from build123d import *

# Parameters (mm, degrees)
SKETCH1_W            = 60
SKETCH1_H            = 20
BOSS_EXTRUDE1_DEPTH  = 3
FILLET1_R            = 10
SKETCH36_R           = 7.1
BOSS_EXTRUDE15_DEPTH = 2
SKETCH37_R           = 9.2
BOSS_EXTRUDE16_DEPTH = 2
SKETCH39_R           = 7.1
BOSS_EXTRUDE18_DEPTH = 2
SKETCH40_R           = 9.2
BOSS_EXTRUDE19_DEPTH = 2
SKETCH41_R           = 7.1
BOSS_EXTRUDE20_DEPTH = 2
SKETCH42_R           = 4
CUT_EXTRUDE5_DEPTH   = 13
SKETCH43_R           = 2.75
CUT_EXTRUDE6_DEPTH   = 3


with BuildPart() as part:
    # Sketch1 → Boss-Extrude1 (new body)
    with BuildSketch(Plane(origin=(0, 0, 0), x_dir=(1, 0, 0), z_dir=(0, 1, 0))):
        Rectangle(SKETCH1_W, SKETCH1_H)
    extrude(amount=BOSS_EXTRUDE1_DEPTH)

    # Fillet1
    fillet1_edges = [part.edges().sort_by_distance(p)[0] for p in [
        (30, 1.5, -10),
        (30, 1.5, 10),
        (-30, 1.5, 10),
        (-30, 1.5, -10),
    ]]
    fillet(fillet1_edges, radius=FILLET1_R - 0.0001)  # a hair under: the kernel refuses the full size

    # Sketch36 → Boss-Extrude15 (add)
    with BuildSketch(Plane(origin=(0, 3, 0), x_dir=(1, 0, 0), z_dir=(0, 1, 0))):
        with Locations(Location((0, 0, 0), (0, 0, 90))):
            Circle(SKETCH36_R)
    extrude(amount=BOSS_EXTRUDE15_DEPTH)

    # Sketch37 → Boss-Extrude16 (add)
    with BuildSketch(Plane(origin=(0, 5, 0), x_dir=(1, 0, 0), z_dir=(0, 1, 0))):
        with Locations(Location((0, 0, 0), (0, 0, 270))):
            Circle(SKETCH37_R)
    extrude(amount=BOSS_EXTRUDE16_DEPTH)

    # Sketch39 → Boss-Extrude18 (add)
    with BuildSketch(Plane(origin=(0, 7, 0), x_dir=(1, 0, 0), z_dir=(0, 1, 0))):
        with Locations(Location((0, 0, 0), (0, 0, 90))):
            Circle(SKETCH39_R)
    extrude(amount=BOSS_EXTRUDE18_DEPTH)

    # Sketch40 → Boss-Extrude19 (add)
    with BuildSketch(Plane(origin=(0, 9, 0), x_dir=(1, 0, 0), z_dir=(0, 1, 0))):
        with Locations(Location((0, 0, 0), (0, 0, 270))):
            Circle(SKETCH40_R)
    extrude(amount=BOSS_EXTRUDE19_DEPTH)

    # Sketch41 → Boss-Extrude20 (add)
    with BuildSketch(Plane(origin=(0, 11, 0), x_dir=(1, 0, 0), z_dir=(0, 1, 0))):
        with Locations(Location((0, 0, 0), (0, 0, 90))):
            Circle(SKETCH41_R)
    extrude(amount=BOSS_EXTRUDE20_DEPTH)

    # Sketch42 → Cut-Extrude5 (cut)
    with BuildSketch(Plane(origin=(0, 13, 0), x_dir=(1, 0, 0), z_dir=(0, 1, 0))):
        with Locations(Location((0, 0, 0), (0, 0, 270))):
            Circle(SKETCH42_R)
    extrude(amount=-CUT_EXTRUDE5_DEPTH, mode=Mode.SUBTRACT)

    # Sketch43 → Cut-Extrude6 (cut)
    with BuildSketch(Plane(origin=(0, 3, 0), x_dir=(1, 0, 0), z_dir=(0, 1, 0))):
        with Locations(Location((-20, 0, 0), (0, 0, 270))):
            Circle(SKETCH43_R)
        with Locations(Location((20, 0, 0), (0, 0, 270))):
            Circle(SKETCH43_R)
    extrude(amount=-CUT_EXTRUDE6_DEPTH, mode=Mode.SUBTRACT)


solid = part.part
Model file for the job. Use its own axes, mm. A direction names the side the tool comes from. Give positions to 0.01 mm unless a question says otherwise; leave off trailing zeros. Loops run counter-clockwise (first coordinate to the right, second up) from the corner with the lowest first, then second, coordinate; pieces in that order, holes last.
1) Saw through at C-C (z = -5.5). Write the cut outline in (x, y), plus the area to 3 significant figures.
2) Saw through at D-D (z = -8). Write the cut outline in (x, y), plus the area to 3 significant figures.
3) Flat gauge pins, fed straight in: pin 1 Ø1.5 at (x, y) = (-5, 7.5) entering from +Z; pin 2 Ø6.5 at (x, z) = (20, 0) entering from +Y; pin 3 Ø4 at (x, z) = (-9.5, -5) entering from +Y. Where does each tip first touch, or does it go through?
4) Saw through at B-B (y = 1.75). Count the separate pieces of the cut face and the enclosed holes in it, plus the area to 3 significant figures.
5) Tool access for faces 4 (the cylindrical face through (2.763, 5.986, 8.775)), 5 (the cylindrical face through (-5.987, 3.986, -3.817)), 6 (the cylindrical face through (27.15, 1.52, -6.99)): list every direction of +Z, -Z, +X, -X, +Y, -Y with a clear straight run to the whole face (end or side of a thin tool).
6) Pull direction Y, two halves, no side cores. Call faces 1 (the flat face through (0, 0, -5)), 2 (the flat face through (0, 1, 10)), 3 (the cylindrical face through (-5.987, 7.986, -3.817)): +Y half, -Y half, draft (parallel to the pull), parting line (faces both ways), or undercut.
7) Wall check: line 1 (X direction, y = 1.4, z = 0); line 2 (Y direction, x = -8, z = -1.5); line 3 (X direction, y = 6, z = 0). Give the ranges that are in metal, low to high.
8) Saw through at A-A (x = 0). Write the cut outline in (y, z).
Answer block:
1. outline: (-28.35, 0) - (28.35, 0) - (28.35, 3) - (4.49, 3) - (4.49, 5) - (7.37, 5) - (7.37, 7) - (4.49, 7) - (4.49, 9) - (7.37, 9) - (7.37, 11) - (4.49, 11) - (4.49, 13) - (-4.49, 13) - (-4.49, 11) - (-7.37, 11) - (-7.37, 9) - (-4.49, 9) - (-4.49, 7) - (-7.37, 7) - (-7.37, 5) - (-4.49, 5) - (-4.49, 3) - (-28.35, 3) - close
1. area: 283 mm2
2. outline: (-26, 0) - (26, 0) - (26, 3) - (-26, 3) - close; (-4.54, 5) - (4.54, 5) - (4.54, 7) - (-4.54, 7) - close; (-4.54, 9) - (4.54, 9) - (4.54, 11) - (-4.54, 11) - close
2. area: 192 mm2
3. pin 1: stops at z = 8.06
3. pin 2: stops at y = 3
3. pin 3: stops at y = 11
4. separate pieces: 1
4. enclosed holes: 3
4. area: 1,020 mm2
5. face 4: +Y
5. face 5: none
5. face 6: -Z, +X, +Y, -Y
6. face 1: -Y half
6. face 2: draft
6. face 3: undercut
7. line 1: x = -30 to -22.75, -17.25 to -4, 4 to 17.25, 22.75 to 30
7. line 2: y = 0 to 3, 5 to 7, 9 to 11
7. line 3: x = -9.2 to -4, 4 to 9.2
8. outline: (0, -10) - (3, -10) - (3, -7.1) - (5, -7.1) - (5, -9.2) - (7, -9.2) - (7, -7.1) - (9, -7.1) - (9, -9.2) - (11, -9.2) - (11, -7.1) - (13, -7.1) - (13, -4) - (0, -4) - close; (0, 4) - (13, 4) - (13, 7.1) - (11, 7.1) - (11, 9.2) - (9, 9.2) - (9, 7.1) - (7, 7.1) - (7, 9.2) - (5, 9.2) - (5, 7.1) - (3, 7.1) - (3, 10) - (0, 10) - close
